Could you check a few things on this model? Use its own coordinates, in mm. A direction names the side the tool comes from. Round coordinates to 2 decimals unless told otherwise and drop trailing zeros. Write each loop counter-clockwise with the first axis right and the second up, starting at its lowest first coordinate (ties: lowest second). Pieces come first, ordered by that corner, then holes. Notation, with made-up numbers: (77.5, 55) -> (131.5, 55) arc R24 cw to (131.5, 68) -> close; hole circle Ø3 at (10.5, -13.5). An arc over 180 degrees is marked (long way). Answer in a Markdown table with one row per item.
from build123d import *

# Parameters (mm, degrees)
SKETCH4_W               = 20
SKETCH4_H               = 30
BOSS_EXTRUDE2_DEPTH     = 16
CUT_EXTRUDE2_DEPTH      = 37.728735344
CUT_EXTRUDE2_DEPTH_BACK = 32
CUT_EXTRUDE4_DEPTH      = 30.681644159
CUT_EXTRUDE4_DEPTH_BACK = 30.681644159
SKETCH7_R               = 2.5
CUT_EXTRUDE5_DEPTH      = 30.681644159
FILLET2_R               = 5
FILLET3_R               = 5
FILLET4_R               = 5
FILLET5_R               = 5
CUT_EXTRUDE6_REACH      = 37.44
SKETCH8_R               = 3.5


with BuildPart() as part:
    # Sketch4 → Boss-Extrude2 (new, symmetric)
    with BuildSketch(Plane(origin=(0, 0, 0), x_dir=(0, 0, -1), z_dir=(1, 0, 0))):
        Rectangle(SKETCH4_W, SKETCH4_H)
    extrude(amount=BOSS_EXTRUDE2_DEPTH, both=True)

    # Sketch5 → Cut-Extrude2 (cut, two sides: drawn at the far end of the back side and taken through both)
    with BuildSketch(Plane.ZY.offset(16).offset(-CUT_EXTRUDE2_DEPTH_BACK)):
        Polygon((-9, -96.021123618), (-9, -15), (-9, 0), (-9, 12), (9, 12), (9, 0), (9, -15), (9, -96.021123618), (9, -258.063370855), (-9, -258.063370855), align=None)
    extrude(amount=CUT_EXTRUDE2_DEPTH + CUT_EXTRUDE2_DEPTH_BACK, mode=Mode.SUBTRACT)

    # Sketch6 → Cut-Extrude4 (cut, two sides: drawn at the far end of the back side and taken through both)
    with BuildSketch(Plane(origin=(0, 0, -10), x_dir=(-1, 0, 0), z_dir=(0, 0, -1)).offset(-CUT_EXTRUDE4_DEPTH_BACK)):
        Polygon((-79.686136493, 80.781027412), (-16, 12), (9, -15), (72.686136493, -83.781027412), (-64.875918332, -211.153300398), (-217.248191317, -46.591245573), align=None)
    extrude(amount=CUT_EXTRUDE4_DEPTH + CUT_EXTRUDE4_DEPTH_BACK, mode=Mode.SUBTRACT)

    # Sketch7 → Cut-Extrude5 (cut, through all)
    with BuildSketch(Plane(origin=(0, 0, -10), x_dir=(-1, 0, 0), z_dir=(0, 0, -1))):
        with Locations((11, -10)):
            Circle(SKETCH7_R)
    extrude(amount=-CUT_EXTRUDE5_DEPTH, mode=Mode.SUBTRACT)

    # Fillet2
    fillet2_edges = [part.edges().sort_by_distance(p)[0] for p in [
        (-16, -15, -9.5),
    ]]
    fillet(fillet2_edges, radius=FILLET2_R)

    # Fillet3
    # the kernel refuses this fillet: 5 mm, written as the material it takes off along each edge
    with BuildSketch(Plane(origin=(-9, -15, -15.449426147), x_dir=(-1, 0, 0), z_dir=(0, 0, 1))) as fillet3_piece_1:
        with BuildLine():
            CenterArc((2.187849813, -4.996469999), FILLET3_R, 92.15310702, 45.049491141)
            Line((-1.480953557, -1.599429841), (-1.554329624, -1.531489038))
            Line((-1.554329624, -1.531489038), (-0.073376067, 0.067940803))
            Line((-0.073376067, 0.067940803), (0, 0.1))
            ThreePointArc((0, 0.1), (1, 0.1), (1.996243004, 0.0999294))
            Line((1.996243004, 0.0999294), (2, 0))
        make_face()
    extrude(amount=11.898852295, mode=Mode.SUBTRACT)

    # Fillet4
    fillet4_edges = [part.edges().sort_by_distance(p)[0] for p in [
        (-16, -15, 9.5),
    ]]
    fillet(fillet4_edges, radius=FILLET4_R)

    # Fillet5
    # the kernel refuses this fillet: 5 mm, written as the material it takes off along each edge
    with BuildSketch(Plane(origin=(-9, -15, 3.550573853), x_dir=(-1, 0, 0), z_dir=(0, 0, 1))) as fillet5_piece_1:
        with BuildLine():
            CenterArc((2.187849813, -4.996469999), FILLET5_R, 92.15310702, 45.049491141)
            Line((-1.480953557, -1.599429841), (-1.554329624, -1.531489038))
            Line((-1.554329624, -1.531489038), (-0.073376067, 0.067940803))
            Line((-0.073376067, 0.067940803), (0, 0.1))
            ThreePointArc((0, 0.1), (1, 0.1), (1.996243004, 0.0999294))
            Line((1.996243004, 0.0999294), (2, 0))
        make_face()
    extrude(amount=11.898852295, mode=Mode.SUBTRACT)

    # Sketch8 → Cut-Extrude6 (cut, up to next)
    with BuildSketch(Plane(origin=(0, 15, 0), x_dir=(1, 0, 0), z_dir=(0, 1, 0)), mode=Mode.PRIVATE) as cut_extrude6_sk1:
        with Locations(Location((4, 0, 0), (0, 0, 270))):
            Circle(SKETCH8_R)
    cut_extrude6_tool1 = extrude(cut_extrude6_sk1.sketch, amount=-CUT_EXTRUDE6_REACH, mode=Mode.PRIVATE) & part.part
    add(cut_extrude6_tool1.solids().sort_by_distance((4, 15, 0))[0], mode=Mode.SUBTRACT)


solid = part.part
1) Imagine slicing it at A-A, the plane z = 0. Please give me the cut outline in (x, y), plus the area to 3 significant figures.
Findings:
| item | result |
|---|---|
| outline | (-16, 12) -> (0.5, 12) -> (0.5, 15) -> (-16, 15) -> close; (7.5, 12) -> (16, 12) -> (16, 15) -> (7.5, 15) -> close |
| area | 75.0 mm^2 |
2) For pin 1 (5 mm diameter, centred on x = 8.5, y = -2, fed in from +Z), with a flat end and sliding along its axis, tell me the tip position at first contact or that it passes through.
Findings:
| item | result |
|---|---|
| pin 1 | passes through |
3) Imagine slicing it at C-C, the plane y = 11.5. Please give me the cut outline in (x, z).
Findings:
| item | result |
|---|---|
| outline | (-16, -10) -> (15.54, -10) -> (15.54, -9) -> (-16, -9) -> close; (-16, 9) -> (15.54, 9) -> (15.54, 10) -> (-16, 10) -> close |
4) Imagine slicing it at D-D, the plane y = -11.5. Please give me the cut outline in (x, z).
Findings:
| item | result |
|---|---|
| outline | (-15.77, -10) -> (-13, -10) -> (-13, -9) -> (-15.77, -9) -> close; (-15.77, 9) -> (-13, 9) -> (-13, 10) -> (-15.77, 10) -> close; (-9, -10) -> (-5.76, -10) -> (-5.76, -9) -> (-9, -9) -> close; (-9, 9) -> (-5.76, 9) -> (-5.76, 10) -> (-9, 10) -> close |
5) Thinking about a two-plate mould opening in X: for faces 3 (the face through (-10.46, -12.44, -9.51)), 4 (the face through (16, 14, 0)), 5 (the face through (0, 15, 0)), which applies, +X half, -X half, draft (parallel to the pull), parting line (faces both ways), or undercut?
Findings:
| item | result |
|---|---|
| face 3 | undercut |
| face 4 | +X half |
| face 5 | draft |
6) Imagine slicing it at B-B, the plane x = 4. Please give me the cut outline in (y, z).
Findings:
| item | result |
|---|---|
| outline | (-0.96, -10) -> (15, -10) -> (15, -3.5) -> (12, -3.5) -> (12, -9) -> (-0.96, -9) -> close; (-0.96, 9) -> (12, 9) -> (12, 3.5) -> (15, 3.5) -> (15, 10) -> (-0.96, 10) -> close |
7) For faces 1 (the face through (4.41, -0.52, -9.49)), 2 (the face through (0, 12, 0)), which set-ups out of +Z, -Z, +X, -X, +Y, -Y let a thin tool reach every point of the face, with its end or its side?
Findings:
| item | result |
|---|---|
| face 1 | +Z, -Z, +X, -Y |
| face 2 | +X, -X, -Y |
8) Please list where these lines run through material, in increasing order: line 1 (Z direction, x = -8.5, y = 4.5); line 2 (Y direction, x = -11, z = 9.7); line 3 (X direction, y = 14.05, z = 0).
Findings:
| item | result |
|---|---|
| line 1 | z = -10 to -9, 9 to 10 |
| line 2 | y = -15 to -12.5, -7.5 to 15 |
| line 3 | x = -16 to 0.5, 7.5 to 16 |
